from build123d import *

# Parameters (mm, degrees)
SKETCH2_R           = 1.5
SKETCH2_W           = 6.488584399
SKETCH2_H           = 3.846601045
BOSS_EXTRUDE2_DEPTH = 1.5


with BuildPart() as part:
    # Sketch2 → Boss-Extrude2 (new body)
    with BuildSketch(Plane(origin=(0, 0, 0), x_dir=(1, 0, 0), z_dir=(0, 1, 0))):
        with BuildLine():
            ThreePointArc((23.247996545, -19.500190875), (24.776607327, -21.890134515), (24.695421013, -24.725957202))
            ThreePointArc((24.695421013, -24.725957202), (21.863295263, -24.863949953), (19.264117039, -25.997197864))
            ThreePointArc((19.264117039, -25.997197864), (0, -34.136214734), (-19.264117039, -25.997197864))
            ThreePointArc((-19.264117039, -25.997197864), (-21.863295263, -24.863949953), (-24.695421013, -24.725957202))
            ThreePointArc((-24.695421013, -24.725957202), (-24.776607327, -21.890134515), (-23.247996545, -19.500190875))
            ThreePointArc((-23.247996545, -19.500190875), (-17.299915505, -0.254242625), (-22.945369046, 19.082640433))
            ThreePointArc((-22.945369046, 19.082640433), (-25.316903499, 21.537699802), (-25.294419588, 24.951053966))
            ThreePointArc((-25.294419588, 24.951053966), (-22.344172838, 24.887982121), (-19.582319286, 25.927260189))
            ThreePointArc((-19.582319286, 25.927260189), (-0.66060428, 33.9728721), (18.359891541, 26.163652643))
            ThreePointArc((18.359891541, 26.163652643), (21.442039723, 24.947145004), (24.750195634, 25.135911308))
            ThreePointArc((24.750195634, 25.135911308), (24.924707249, 21.788182903), (22.945369046, 19.082640433))
            ThreePointArc((22.945369046, 19.082640433), (17.299915505, -0.254242625), (23.247996545, -19.500190875))
        make_face()
        with Locations(Location((-15.25, 15.25, 0), (0, 0, 270))):
            Circle(SKETCH2_R, mode=Mode.SUBTRACT)
        with Locations(Location((15.25, 15.25, 0), (0, 0, 270))):
            Circle(SKETCH2_R, mode=Mode.SUBTRACT)
        with Locations(Location((-15.25, -15.25, 0), (0, 0, 270))):
            Circle(SKETCH2_R, mode=Mode.SUBTRACT)
        with Locations(Location((15.25, -15.25, 0), (0, 0, 270))):
            Circle(SKETCH2_R, mode=Mode.SUBTRACT)
        with Locations(Location((-22.519911508, 22.116468281, 0), (0, 0, 270))):
            Circle(SKETCH2_R, mode=Mode.SUBTRACT)
        with Locations(Location((22.519911508, 22.116468281, 0), (0, 0, 270))):
            Circle(SKETCH2_R, mode=Mode.SUBTRACT)
        with Locations(Location((22.519911508, -22.116468281, 0), (0, 0, 270))):
            Circle(SKETCH2_R, mode=Mode.SUBTRACT)
        with Locations(Location((-22.519911508, -22.116468281, 0), (0, 0, 270))):
            Circle(SKETCH2_R, mode=Mode.SUBTRACT)
        with Locations((3.2442922, -27.038937624)):
            Rectangle(SKETCH2_W, SKETCH2_H, mode=Mode.SUBTRACT)
    extrude(amount=BOSS_EXTRUDE2_DEPTH)


solid = part.part
Verification items for the finished model (mm, model axes). A direction names the side the tool comes from. Give positions to 0.01 mm unless a question says otherwise; leave off trailing zeros. Loops run counter-clockwise (first coordinate to the right, second up) from the corner with the lowest first, then second, coordinate; pieces in that order, holes last. Notation, with made-up numbers: (31, 55) - (44, 55) arc R10 ccw to (44, 62) - close; hole circle Ø5 at (20.25, 39). An arc over 180 degrees is marked (long way). Write each question's results on one line, items separated by ' | '.
1) Sectioned sample at A-A on x = 15.25. Record the boundary of the cut face in (y, z).
Solution:
outline: (0, -28.83) - (1.5, -28.83) - (1.5, -16.75) - (0, -16.75) - close; (0, -13.75) - (1.5, -13.75) - (1.5, 13.75) - (0, 13.75) - close; (0, 16.75) - (1.5, 16.75) - (1.5, 29.39) - (0, 29.39) - close
2) Sectioned sample at B-B on z = 27. Record the boundary of the cut face in (x, y), plus the area to 3 significant figures.
Solution:
outline: (-18.24, 0) - (0, 0) - (0, 1.5) - (-18.24, 1.5) - close; (6.49, 0) - (18.24, 0) - (18.24, 1.5) - (6.49, 1.5) - close | area: 45.0 mm2
3) Sectioned sample at D-D on z = 15.25. Record the boundary of the cut face in (x, y).
Solution:
outline: (-20.81, 0) - (-16.75, 0) - (-16.75, 1.5) - (-20.81, 1.5) - close; (-13.75, 0) - (13.75, 0) - (13.75, 1.5) - (-13.75, 1.5) - close; (16.75, 0) - (20.81, 0) - (20.81, 1.5) - (16.75, 1.5) - close
4) Tool access check on faces 1 (the flat face through (3, 1, 25.116)), 2 (the cylindrical face through (24.766, 0.74, 21.851)). Record the directions out of +Z, -Z, +X, -X, +Y, -Y that give a thin tool (end or side, any length) a straight path to the whole face; none if there is none.
Solution:
face 1: +Y, -Y | face 2: +X, +Y, -Y
5) Depth check by flat-ended pin: P1, Ø0.8, axis at y = 1, z = 27, coming from the -X side. Enter the tip coordinate at first touch or a pass-through.
Solution:
P1: x = -18.66
6) Sectioned sample at C-C on y = 0.45. Count the separate pieces of the cut face and the enclosed holes in it, plus the area to 3 significant figures.
Solution:
separate pieces: 1 | enclosed holes: 9 | area: 2,460 mm2
7) Material ranges on L1, parallel to Z at x = -16, y = 0.9; L2, parallel to X at y = 0.85, z = -15.25; L3, parallel to Z at x = 4, y = 0.1, recorded low to high. Write a range as from..to.
Solution:
L1: -29..-16.55, -13.95..13.95, 16.55..28.85 | L2: -20.79..-16.75, -13.75..13.75, 16.75..20.79 | L3: -33.59..25.12, 28.96..33.84
8) Mould release check, pull along X, two halves, no side actions. Record for faces 3 (the cylindrical face through (-15.18, 0.74, 13.75)), 4 (the cylindrical face through (0.301, 0.74, 34.135)), 5 (the cylindrical face through (17.3, 0.7, 0)), 6 (the cylindrical face through (21.396, 0.74, -24.955)): pulls with the +X half, pulls with the -X half, needs draft (parallel to the pull), parting line crosses it, or undercut.
Solution:
face 3: undercut | face 4: parting line crosses it | face 5: pulls with the +X half | face 6: undercut
